from build123d import *

# Parameters (mm, degrees)
BOSS_EXTRUDE1_DEPTH = 50
SKETCH2_R           = 7.5
CUT_EXTRUDE1_DEPTH  = 104.07764064
FILLET1_R           = 30
FILLET2_R           = 30


with BuildPart() as part:
    # Sketch1 → Boss-Extrude1 (new, symmetric)
    with BuildSketch(Plane.XY):
        Polygon((0, 0), (-75, 0), (-75, 40), (25, 40), (25, 10), (75, 10), (75, 0), align=None)
    boss_extrude1 = extrude(amount=BOSS_EXTRUDE1_DEPTH, both=True)

    # Mirror1: Boss-Extrude1 across plane
    add(boss_extrude1.mirror(Plane(origin=(0, 0, -50), x_dir=(0, 0, 1), z_dir=(0, -1, 0))))

    # Sketch2 → Cut-Extrude1 (cut, through all)
    with BuildSketch(Plane(origin=(0, 10, 0), x_dir=(1, 0, 0), z_dir=(0, 1, 0))):
        with Locations(Location((60, 0, 0), (0, 0, 270))):
            Circle(SKETCH2_R)
    extrude(amount=-CUT_EXTRUDE1_DEPTH, mode=Mode.SUBTRACT)

    # Fillet1
    fillet1_edges = [part.edges().sort_by_distance(p)[0] for p in [
        (75, 0, -50),
    ]]
    fillet(fillet1_edges, radius=FILLET1_R)

    # Fillet2
    fillet2_edges = [part.edges().sort_by_distance(p)[0] for p in [
        (75, 0, 50),
    ]]
    fillet(fillet2_edges, radius=FILLET2_R)


solid = part.part
Geometry check sheet. Reference: the model listing, model coordinates, mm. A direction names the side the tool comes from. Give positions to 0.01 mm unless a question says otherwise; leave off trailing zeros. Loops run counter-clockwise (first coordinate to the right, second up) from the corner with the lowest first, then second, coordinate; pieces in that order, holes last.
(1) Section check D-D on y = -24. Record the cut outline in (x, z).
From the geometry:
outline: (-75, -50) - (25, -50) - (25, 50) - (-75, 50) - close
(2) Set-up check for faces 1 (the flat face through (25, 25, 1)), 2 (the flat face through (-26, -40, 1)), 3 (the flat face through (25, -25, 1)): record each of +Z, -Z, +X, -X, +Y, -Y from which the full face is reachable in a straight line by a thin tool's end or side.
From the geometry:
face 1: +Z, -Z, +X, +Y
face 2: +Z, -Z, +X, -X, -Y
face 3: +Z, -Z, +X, -Y
(3) Release check for a two-part mould opening along X. For faces 4 (the cylindrical face through (67.436, 0.14, -0.976)), 5 (the flat face through (-75, 1, 1)), 6 (the flat face through (-26, 40, 1)) record: released by +X, released by -X, zero draft, split by the parting line, or undercut.
From the geometry:
face 4: undercut
face 5: released by -X
face 6: zero draft
(4) Depth check by flat-ended pin: pin 1 Ø9 at (x, z) = (60, 0) entering from -Y; pin 2 Ø12 at (x, z) = (38, 35.5) entering from -Y; pin 3 Ø15 at (y, z) = (22.5, 19.5) entering from +X. Enter the tip coordinate at first touch or a pass-through.
From the geometry:
pin 1: passes through
pin 2: stops at y = -10
pin 3: stops at x = 25
(5) Section check A-A on z = 0. Record the cut outline in (x, y).
From the geometry:
outline: (-75, -40) - (25, -40) - (25, -10) - (52.5, -10) - (52.5, 10) - (25, 10) - (25, 40) - (-75, 40) - close; (67.5, -10) - (75, -10) - (75, 10) - (67.5, 10) - close
(6) Section check C-C on z = 30. Record the cut outline in (x, y), then the cut area to 3 significant figures.
From the geometry:
outline: (-75, -40) - (25, -40) - (25, -10) - (73.28, -10) - (73.28, 10) - (25, 10) - (25, 40) - (-75, 40) - close
area: 8,970 mm2
(7) Thickness scan on L1, parallel to X at y = -4, z = 0; L2, parallel to X at y = -16, z = -28; L3, parallel to Y at x = 34, z = 23. Record the ranges inside material, lowest first.
From the geometry:
L1: x = -75 to 52.5, 67.5 to 75
L2: x = -75 to 25
L3: y = -10 to 10
(8) Section check B-B on x = 60. Record the cut outline in (y, z).
From the geometry:
outline: (-10, -45.98) - (10, -45.98) - (10, -7.5) - (-10, -7.5) - close; (-10, 7.5) - (10, 7.5) - (10, 45.98) - (-10, 45.98) - close
